Geometry: see drawing. Coordinates: mm, zero at the bounding-box minimum. Coordinates: 2 decimals unless noted, no trailing zeros. Write each loop counter-clockwise with the first axis right and the second up, starting at its lowest first coordinate (ties: lowest second). Pieces come first, ordered by that corner, then holes.
1) Line query: L1, parallel to Z at x = 6, y = 1; L2, parallel to X at y = 1.3, z = 56; L3, parallel to Z at x = 35.5, y = 1.55. Output: solid intervals per line, ascending.
2) Section query B-B (x = 33). Output: boundary loops of the cut face in (y, z).
3) Section query A-A (y = 1.15). Output: boundary loops of the cut face in (x, z).
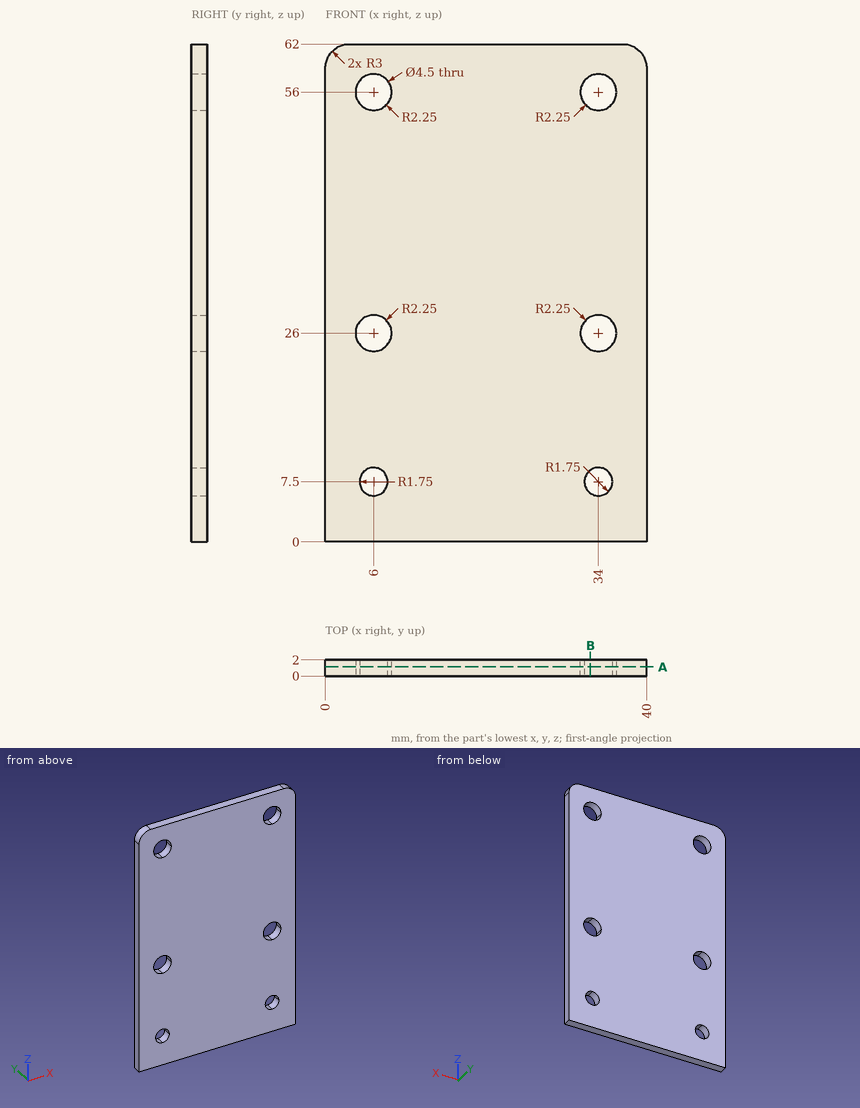
Answer:
1. L1: z = 0 to 5.75, 9.25 to 23.75, 28.25 to 53.75, 58.25 to 62
1. L2: x = 0 to 3.75, 8.25 to 31.75, 36.25 to 40
1. L3: z = 0 to 6.6, 8.4 to 24.32, 27.68 to 54.32, 57.68 to 62
2. outline: (0, 0) - (2, 0) - (2, 6.06) - (0, 6.06) - close; (0, 8.94) - (2, 8.94) - (2, 23.98) - (0, 23.98) - close; (0, 28.02) - (2, 28.02) - (2, 53.98) - (0, 53.98) - close; (0, 58.02) - (2, 58.02) - (2, 62) - (0, 62) - close
3. outline: (0, 0) - (40, 0) - (40, 59) arc R3 ccw to (37, 62) - (3, 62) arc R3 ccw to (0, 59) - close; hole circle Ø4.5 at (6, 26); hole circle Ø4.5 at (6, 56); hole circle Ø3.5 at (6, 7.5); hole circle Ø4.5 at (34, 26); hole circle Ø4.5 at (34, 56); hole circle Ø3.5 at (34, 7.5)
